```python
from build123d import *

# Parameters (mm, degrees)
CROQUIS1_W              = 20
CROQUIS1_H              = 35
CROQUIS1_R              = 5
SALIENTE_EXTRUIR1_DEPTH = 20
CROQUIS2_R              = 2
SALIENTE_EXTRUIR2_DEPTH = 8
CROQUIS3_W              = 20
CROQUIS3_H              = 20
SALIENTE_EXTRUIR3_DEPTH = 10
CORTAR_EXTRUIR1_REACH   = 442.837
CROQUIS4_R              = 0.5
SALIENTE_EXTRUIR4_START = 12.5
CROQUIS5_W              = 20
CROQUIS5_H              = 12
CROQUIS5_R              = 0.5
SALIENTE_EXTRUIR4_DEPTH = 12.5
CROQUIS6_R              = 5.5
CORTAR_EXTRUIR2_DEPTH   = 441.837042541
CROQUIS7_W              = 11
CROQUIS7_H              = 11
CORTAR_EXTRUIR3_DEPTH   = 18
CROQUIS8_W              = 16
CROQUIS8_H              = 13.5
CORTAR_EXTRUIR4_DEPTH   = 1.5


with BuildPart() as part:
    # Croquis1 → Saliente-Extruir1 (new body)
    with BuildSketch(Plane(origin=(0, 0, 0), x_dir=(1, 0, 0), z_dir=(0, 1, 0))):
        with Locations((-428.226450018, 26.030180121)):
            Rectangle(CROQUIS1_W, CROQUIS1_H)
        with Locations(Location((-428.226450018, 18.530180121, 0), (0, 0, 270))):
            Circle(CROQUIS1_R, mode=Mode.SUBTRACT)
        with Locations(Location((-428.226450018, 33.530180121, 0), (0, 0, 270))):
            Circle(CROQUIS1_R, mode=Mode.SUBTRACT)
    extrude(amount=SALIENTE_EXTRUIR1_DEPTH)

    # Croquis2 → Saliente-Extruir2 (add)
    with BuildSketch(Plane(origin=(-418.226450018, 0, 0), x_dir=(0, 0, -1), z_dir=(1, 0, 0))):
        with Locations(Location((18.530180121, 12.2, 0), (0, 0, 180))):
            Circle(CROQUIS2_R)
    extrude(amount=SALIENTE_EXTRUIR2_DEPTH)

    # Croquis3 → Saliente-Extruir3 (add)
    with BuildSketch(Plane.XY.offset(-8.530180121)):
        with Locations((-428.226450018, 10)):
            Rectangle(CROQUIS3_W, CROQUIS3_H)
    extrude(amount=SALIENTE_EXTRUIR3_DEPTH)

    # Croquis4 → Cortar-Extruir1 (cut, up to next)
    with BuildSketch(Plane(origin=(0, 20, 0), x_dir=(1, 0, 0), z_dir=(0, 1, 0)), mode=Mode.PRIVATE) as cortar_extruir1_sk1:
        with Locations(Location((-428.226450018, 4.530180121, 0), (0, 0, 270))):
            Circle(CROQUIS4_R)
    cortar_extruir1_tool1 = extrude(cortar_extruir1_sk1.sketch, amount=-CORTAR_EXTRUIR1_REACH, mode=Mode.PRIVATE) & part.part
    add(cortar_extruir1_tool1.solids().sort_by_distance((-428.22645, 20, -4.53018))[0], mode=Mode.SUBTRACT)

    # Croquis5 → Saliente-Extruir4 (add)
    with BuildSketch(Plane(origin=(0, 20, 0), x_dir=(1, 0, 0), z_dir=(0, 1, 0)).offset(SALIENTE_EXTRUIR4_START)):
        with Locations((-428.226450018, 4.530180121)):
            Rectangle(CROQUIS5_W, CROQUIS5_H)
        with Locations(Location((-428.226450018, 4.530180121, 0), (0, 0, 270))):
            Circle(CROQUIS5_R, mode=Mode.SUBTRACT)
    extrude(amount=-SALIENTE_EXTRUIR4_DEPTH)

    # Croquis6 → Cortar-Extruir2 (cut, through all)
    with BuildSketch(Plane(origin=(0, 20, 0), x_dir=(1, 0, 0), z_dir=(0, 1, 0))):
        with Locations(Location((-428.226450018, 18.530180121, 0), (0, 0, 270))):
            Circle(CROQUIS6_R)
        with Locations(Location((-428.226450018, 33.530180121, 0), (0, 0, 270))):
            Circle(CROQUIS6_R)
    extrude(amount=-CORTAR_EXTRUIR2_DEPTH, mode=Mode.SUBTRACT)

    # Croquis7 → Cortar-Extruir3 (cut)
    with BuildSketch(Plane(origin=(-410.226450018, 0, 0), x_dir=(0, 0, -1), z_dir=(1, 0, 0))):
        with Locations((18.530180121, 12.2)):
            Rectangle(CROQUIS7_W, CROQUIS7_H)
    extrude(amount=-CORTAR_EXTRUIR3_DEPTH, mode=Mode.SUBTRACT)

    # Croquis8 → Cortar-Extruir4 (cut)
    with BuildSketch(Plane(origin=(-418.226450018, 0, 0), x_dir=(0, 0, -1), z_dir=(1, 0, 0))):
        with Locations((18.530180121, 10.95)):
            Rectangle(CROQUIS8_W, CROQUIS8_H)
    extrude(amount=-CORTAR_EXTRUIR4_DEPTH, mode=Mode.SUBTRACT)


solid = part.part
```
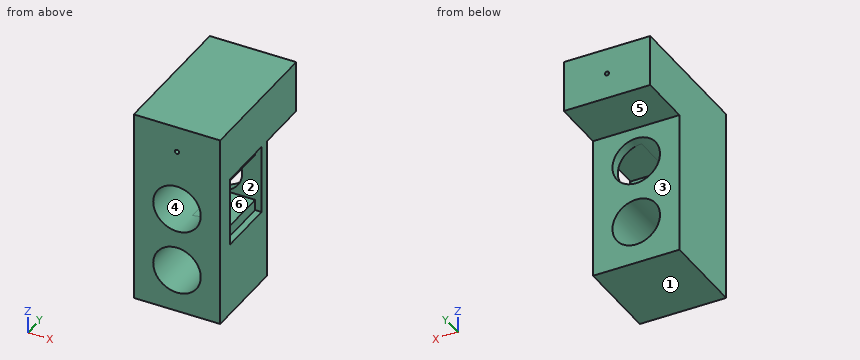
Geometry: final body of the model. Coordinates: model frame, mm. Face numbers are marked on the shaded views. A direction names the side the tool comes from. Coordinates: 2 decimals unless noted, no trailing zeros. Write each loop counter-clockwise with the first axis right and the second up, starting at its lowest first coordinate (ties: lowest second). Pieces come first, ordered by that corner, then holes. Notation, with made-up numbers: M -7.5,78.25 L 26.5,78.25 A15 cw 26.5,93.25 Z; hole C -31,-21 d11. An arc over 180 degrees is marked long. Answer as CSV lines item,"result". Start each with the question number.
Q1. Cut plane C-C on x = -433. Return the cut outline in (y, z), then the cut area to 3 significant figures.
Q2. Mould query, pull axis Y, two halves, no side actions, for the marked faces 1, 2 and 3. Classes: released by +Y, released by -Y, zero draft, split by the parting line, or undercut.
Q3. Cut plane A-A on y = 11. Return the cut outline in (x, z).
Q4. Pin query (flat end, axial travel): P1, Ø0.8, axis at x = -419, z = -17, coming from the +Y side; P2, Ø10, axis at x = -424, y = 27, coming from the -Z side; P3, Ø10, axis at x = -428.23, z = -33.53, coming from the +Y side. Return the tip coordinate at first contact, or that it passes through.
Q5. Line query: line 1 (Z direction, x = -420, y = 14); line 2 (Z direction, x = -425.5, y = 12.5); line 3 (Z direction, x = -425.5, y = 4.5). Output: solid intervals per line, ascending. Write a range as from..to.
Q6. Cut plane D-D on z = -25.5. Return the cut outline in (x, y), then the cut area to 3 significant figures.
Q7. Cut plane B-B on y = 2.5. Return the cut outline in (x, z).
Q8. Reachability of the marked faces 4, 5 and 6 from +Z, -Z, +X, -X, +Y, -Y: full face, straight path, thin tool, end or side. Return the list, or none.
Findings below:
1,outline,"M 0,-43.53 L 20,-43.53 L 20,-36.26 L 0,-36.26 Z; M 0,-30.8 L 20,-30.8 L 20,-21.26 L 0,-21.26 Z; M 0,-15.8 L 20,-15.8 L 20,-10.53 L 32.5,-10.53 L 32.5,1.47 L 0,1.47 Z"
1,area,"831 mm2"
2,face 1,"zero draft"
2,face 2,"undercut"
2,face 3,"released by +Y"
3,outline,"M -438.23,-43.53 L -418.23,-43.53 L -418.23,-26.53 L -419.73,-26.53 L -419.73,-24.03 L -428.23,-24.03 A5.5 cw -428.23,-13.03 L -419.73,-13.03 L -419.73,-10.53 L -418.23,-10.53 L -418.23,1.47 L -438.23,1.47 Z; hole C -428.23,-33.53 d11; hole C -428.23,-4.53 d1"
4,P1,"stops at y = 20"
4,P2,"stops at z = -10.53"
4,P3,"passes through"
5,line 1,"z = -43.53..-24.03, -13.03..1.47"
5,line 2,"z = -43.53..-38.31, -28.75..-24.03, -13.03..1.47"
5,line 3,"z = -43.53..-38.31, -28.75..-23.31, -13.75..1.47"
6,outline,"M -438.23,0 L -418.23,0 L -418.23,4.2 L -419.73,4.2 L -419.73,17.7 L -418.23,17.7 L -418.23,20 L -438.23,20 Z"
6,area,"380 mm2"
7,outline,"M -438.23,-43.53 L -418.23,-43.53 L -418.23,1.47 L -438.23,1.47 Z; hole C -428.23,-33.53 d11; hole C -428.23,-18.53 d11; hole C -428.23,-4.53 d1"
8,face 4,"+Y, -Y"
8,face 5,"-Z, +X, -X, +Y"
8,face 6,"+X"
